Geometry: final body of the model. Coordinates: model frame, mm. Face numbers are marked on the shaded views. A direction names the side the tool comes from. Give positions to 0.01 mm unless a question says otherwise; leave off trailing zeros. Write each loop counter-clockwise with the first axis right and the second up, starting at its lowest first coordinate (ties: lowest second). Pieces come first, ordered by that corner, then holes. Notation, with made-up numbers: M -24,-32.5 L -15,-32.5 A23 ccw -15,3.5 Z; hole C -22,85.25 d3. An arc over 180 degrees is marked long. Use a Markdown table: item, result. Add a question column.
(1) Cut plane B-B (z = 7.75). Output: boundary loops of the cut face in (x, y), plus the area to 3 significant figures.
(2) Cut plane C-C (x = 9). Output: boundary loops of the cut face in (y, z), plus the area to 3 significant figures.
(3) Cut plane A-A (y = 28.5). Output: boundary loops of the cut face in (x, z).
(4) Material intervals for L1, parallel to Z at x = 20, y = -2; L2, parallel to X at y = 2, z = 4.5; L3, parallel to Y at x = -1, z = 12, sorted ascending.
(5) Draft query along Y for the marked faces 1, 2, 3 and 4. Return one class per face: released by +Y, released by -Y, zero draft, split by the parting line, or undercut.
(6) Reachability of the marked faces 5 and 6 from +Z, -Z, +X, -X, +Y, -Y: full face, straight path, thin tool, end or side. Return the list, or none.
(7) Pin query (flat end, axial travel): pin 1 Ø1 at (x, z) = (12.5, 0.5) entering from +Y; pin 2 Ø2 at (x, z) = (24, 2.5) entering from +Y; pin 3 Ø4 at (y, z) = (30, 6.5) entering from +X. Return the tip coordinate at first contact, or that it passes through.
```python
from build123d import *

# Parameters (mm, degrees)
F0_R     = 2.5
F1_DEPTH = 1.2
F2_DEPTH = 15
F3_R     = 3.99999


# Not quite as in the source:
# - a fillet or chamfer is up to 0.001 mm smaller than in the source, because OpenCascade refuses the exact size


with BuildPart() as f1:
    # F0 (on Top) → F1 (new body)
    with BuildSketch(Plane.XY):
        Polygon((4, 34), (-4, 34), (-4, -4), (29, -4), (29, 4), (4, 4), align=None)
        Circle(F0_R, mode=Mode.SUBTRACT)
        with Locations((25, 0)):
            Circle(F0_R, mode=Mode.SUBTRACT)
        with Locations((0, 30)):
            Circle(F0_R, mode=Mode.SUBTRACT)
    extrude(amount=F1_DEPTH)

    # F0 (on Top) → F2 (join)
    with BuildSketch(Plane.XY):
        Circle(F0_R)
        with Locations((25, 0)):
            Circle(F0_R)
        with Locations((0, 30)):
            Circle(F0_R)
    extrude(amount=F2_DEPTH)

    # F3 (radius 4 in the source; OpenCascade refuses exactly that, so slightly less here)
    f3_edges = [f1.edges().sort_by_distance(p)[0] for p in [
        (4, 4, 0.6),
        (29, 4, 0.6),
        (29, -4, 0.6),
        (-4, -4, 0.6),
        (-4, 34, 0.6),
        (4, 34, 0.6),
    ]]
    fillet(f3_edges, radius=F3_R)


solid = f1.part
```
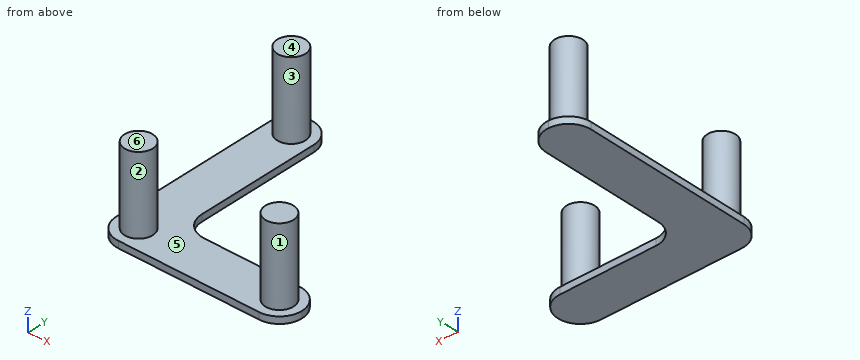
Answer list:
| question | item | result |
|---|---|---|
| 1 | outline | C 0,0 d5; C 0,30 d5; C 25,0 d5 |
| 1 | area | 58.9 mm² |
| 2 | outline | M -4,0 L 4,0 L 4,1.2 L -4,1.2 Z |
| 2 | area | 9.60 mm² |
| 3 | outline | M -4,0 L 4,0 L 4,1.2 L 2,1.2 L 2,15 L -2,15 L -2,1.2 L -4,1.2 Z |
| 4 | L1 | 0 to 1.2 |
| 4 | L2 | -1.5 to 1.5, 23.5 to 26.5 |
| 4 | L3 | -2.29 to 2.29, 27.71 to 32.29 |
| 5 | face 1 | split by the parting line |
| 5 | face 2 | undercut |
| 5 | face 3 | undercut |
| 5 | face 4 | zero draft |
| 6 | face 5 | +Z |
| 6 | face 6 | +Z, +X, -X, +Y, -Y |
| 7 | pin 1 | y = 4 |
| 7 | pin 2 | y = 2.5 |
| 7 | pin 3 | x = 2.5 |
